```python
from build123d import *


with BuildPart() as part:
    # Sketch2 → Revolve2 (revolve)
    with BuildSketch(Plane.XY):
        with BuildLine():
            Line((3, -11), (3, 11))
            Line((3, 11), (7, 11))
            Line((7, 11), (7, 9.5))
            Line((7, 9.5), (22, 9.5))
            ThreePointArc((22, 9.5), (24.121320344, 8.621320344), (25, 6.5))
            Line((25, 6.5), (25, -6.5))
            ThreePointArc((25, -6.5), (24.121320344, -8.621320344), (22, -9.5))
            Line((22, -9.5), (7, -9.5))
            Line((7, -9.5), (7, -11))
            Line((7, -11), (3, -11))
        make_face()
    revolve(axis=Axis((0, 0, 0), (0, 1, 0)))


solid = part.part
```
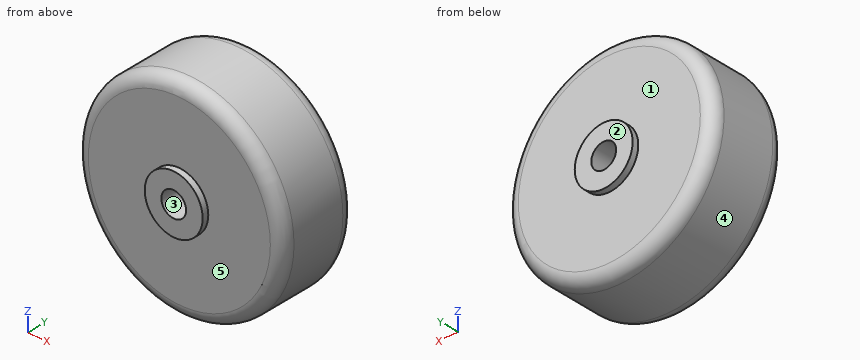
Can you work these out from the model? Positions are in its coordinate system, mm. Face numbers are marked on the shaded views. A direction names the side the tool comes from. Coordinates: 2 decimals unless noted, no trailing zeros. Write each loop counter-clockwise with the first axis right and the second up, starting at its lowest first coordinate (ties: lowest second). Pieces come first, ordered by that corner, then holes. Notation, with made-up numbers: (0, -17.75) - (38, -17.75) arc R27 ccw to (38, -1.75) - close; hole circle Ø9 at (14.25, 83.25). An arc over 180 degrees is marked (long way). Return JSON: item names as keys, results as strings.
Q1. On a 3-axis mill with a long thin cutter (end or side, diameter ignored), from which of +Z, -Z, +X, -X, +Y, -Y can I reach the whole of each face in a straight line? I mean the marked faces 1 and 2. Say none if no direction works.
Computed values:
{"face 1": "+Y", "face 2": "+Z, -Z, +X, -X, +Y"}
Q2. I'm going to push flat-ended pins straight in: pin 1 Ø12 at (y, z) = (7.5, -2) entering from +X; pin 2 Ø12 at (y, z) = (3, 9.5) entering from +X; pin 3 Ø1 at (y, z) = (-1.5, 11) entering from -X; pin 4 Ø10 at (y, z) = (-6, -18) entering from +X. Where does each tip first touch, or does it pass through?
Computed values:
{"pin 1": "stops at x = 25", "pin 2": "stops at x = 24.75", "pin 3": "stops at x = -22.69", "pin 4": "stops at x = 21.35"}
Q3. If we section it at B-B (z = 0): Please give me the cut outline in (x, y).
Computed values:
{"outline": "(-25, -6.5) arc R3 ccw to (-22, -9.5) - (-7, -9.5) - (-7, -11) - (-3, -11) - (-3, 11) - (-7, 11) - (-7, 9.5) - (-22, 9.5) arc R3 ccw to (-25, 6.5) - close; (3, -11) - (7, -11) - (7, -9.5) - (22, -9.5) arc R3 ccw to (25, -6.5) - (25, 6.5) arc R3 ccw to (22, 9.5) - (7, 9.5) - (7, 11) - (3, 11) - close"}
Q4. Please list where these lines run through material, in increasing order: L1, parallel to Z at x = 0, y = -1; L2, parallel to Y at x = 5.5, z = -13. Write a range as from..to.
Computed values:
{"L1": "z = -25..-3, 3..25", "L2": "y = -9.5..9.5"}
Q5. If we section it at C-C (y = -2.75): Please give me the cut outline in (x, z), then the cut area to 3 significant figures.
Computed values:
{"outline": "circle Ø50 at (0, 0); hole circle Ø6 at (0, 0)", "area": "1,940 mm2"}
Q6. Thinking about a two-plate mould opening in Z: for the marked faces 3, 4 and 5, which applies, +Z half, -Z half, draft (parallel to the pull), parting line (faces both ways), or undercut?
Computed values:
{"face 3": "undercut", "face 4": "parting line", "face 5": "draft"}
Q7. If we section it at A-A (x = 0): Please give me the cut outline in (y, z), then the cut area to 3 significant figures.
Computed values:
{"outline": "(-11, -7) - (-9.5, -7) - (-9.5, -22) arc R3 ccw to (-6.5, -25) - (6.5, -25) arc R3 ccw to (9.5, -22) - (9.5, -7) - (11, -7) - (11, -3) - (-11, -3) - close; (-11, 3) - (11, 3) - (11, 7) - (9.5, 7) - (9.5, 22) arc R3 ccw to (6.5, 25) - (-6.5, 25) arc R3 ccw to (-9.5, 22) - (-9.5, 7) - (-11, 7) - close", "area": "852 mm2"}
